from build123d import *

# Parameters (mm, degrees)
SKETCH1_W           = 56
SKETCH1_H           = 28
BOSS_EXTRUDE1_DEPTH = 16
SKETCH2_W           = 52
SKETCH2_H           = 24
CUT_EXTRUDE1_DEPTH  = 8
SKETCH3_W           = 24
SKETCH3_H           = 24
CUT_EXTRUDE2_DEPTH  = 2
SKETCH4_W           = 52
SKETCH4_H           = 2
CUT_EXTRUDE3_DEPTH  = 1
SKETCH5_R           = 6.75
CUT_EXTRUDE4_DEPTH  = 1
CUT_EXTRUDE5_REACH  = 7
SKETCH6_R           = 5
SKETCH7_R           = 6.75
CUT_EXTRUDE6_DEPTH  = 1
SKETCH8_R           = 6.75
CUT_EXTRUDE7_DEPTH  = 1
CUT_EXTRUDE8_DEPTH  = 26


with BuildPart() as part:
    # Sketch1 → Boss-Extrude1 (new body)
    with BuildSketch(Plane(origin=(0, 0, 0), x_dir=(1, 0, 0), z_dir=(0, 1, 0))):
        Rectangle(SKETCH1_W, SKETCH1_H)
    extrude(amount=BOSS_EXTRUDE1_DEPTH)

    # Sketch2 → Cut-Extrude1 (cut)
    with BuildSketch(Plane(origin=(0, 16, 0), x_dir=(1, 0, 0), z_dir=(0, 1, 0))):
        Rectangle(SKETCH2_W, SKETCH2_H)
    extrude(amount=-CUT_EXTRUDE1_DEPTH, mode=Mode.SUBTRACT)

    # Sketch3 → Cut-Extrude2 (cut)
    with BuildSketch(Plane(origin=(0, 8, 0), x_dir=(1, 0, 0), z_dir=(0, 1, 0))):
        Rectangle(SKETCH3_W, SKETCH3_H)
    extrude(amount=-CUT_EXTRUDE2_DEPTH, mode=Mode.SUBTRACT)

    # Sketch4 → Cut-Extrude3 (cut)
    with BuildSketch(Plane(origin=(0, 8, 0), x_dir=(1, 0, 0), z_dir=(0, 1, 0))):
        Rectangle(SKETCH4_W, SKETCH4_H)
    extrude(amount=-CUT_EXTRUDE3_DEPTH, mode=Mode.SUBTRACT)

    # Sketch5 → Cut-Extrude4 (cut)
    with BuildSketch(Plane(origin=(0, 6, 0), x_dir=(1, 0, 0), z_dir=(0, 1, 0))):
        Circle(SKETCH5_R)
    extrude(amount=-CUT_EXTRUDE4_DEPTH, mode=Mode.SUBTRACT)

    # Sketch6 → Cut-Extrude5 (cut, up to next)
    with BuildSketch(Plane(origin=(0, 5, 0), x_dir=(1, 0, 0), z_dir=(0, 1, 0)), mode=Mode.PRIVATE) as cut_extrude5_sk1:
        Circle(SKETCH6_R)
    cut_extrude5_tool1 = extrude(cut_extrude5_sk1.sketch, amount=-CUT_EXTRUDE5_REACH, mode=Mode.PRIVATE) & part.part
    add(cut_extrude5_tool1.solids().sort_by_distance((0, 5, 0))[0], mode=Mode.SUBTRACT)

    # Sketch7 → Cut-Extrude6 (cut)
    with BuildSketch(Plane.XY.offset(14)):
        with Locations((0, 8)):
            Circle(SKETCH7_R)
    extrude(amount=-CUT_EXTRUDE6_DEPTH, mode=Mode.SUBTRACT)

    # Sketch8 → Cut-Extrude7 (cut)
    with BuildSketch(Plane(origin=(0, 0, -14), x_dir=(-1, 0, 0), z_dir=(0, 0, -1))):
        with Locations((0, 8)):
            Circle(SKETCH8_R)
    extrude(amount=-CUT_EXTRUDE7_DEPTH, mode=Mode.SUBTRACT)

    # Sketch9 → Cut-Extrude8 (cut)
    with BuildSketch(Plane.XY.offset(13)):
        with BuildLine():
            Line((-4.582575695, 6), (4.582575695, 6))
            ThreePointArc((4.582575695, 6), (0, 13), (-4.582575695, 6))
        make_face()
    extrude(amount=-CUT_EXTRUDE8_DEPTH, mode=Mode.SUBTRACT)

    # Sketch11 → Cut-Revolve2 (revolve, cut)
    with BuildSketch(Plane(origin=(0, 0, 0), x_dir=(0, 0, -1), z_dir=(1, 0, 0))):
        Polygon((0, 0), (-10, 0), (0, 10), align=None)
    revolve(axis=Axis((0, 10, 0), (0, -1, 0)), mode=Mode.SUBTRACT)


solid = part.part
Design review of the part built by this model. Coordinates are the model's own, in mm. A direction names the side the tool comes from. Give positions to 0.01 mm unless a question says otherwise; leave off trailing zeros. Order: outer loops, then holes, each group sorted by start corner. A loop starts at its lowest first (then second) coordinate and runs counter-clockwise, first axis right, second up. Notation, with made-up numbers: (-24.5, 81) - (17.5, 81) arc R25 cw to (17.5, 95) - close; hole circle Ø7 at (46.25, 52). An arc over 180 degrees is marked (long way). Write item = value, one per line. Start each with the question number.
Q1. Tool access review of faces 5 (the face through (-26, 12, 0)), 6 (the face through (0.879, 14.693, -13.507)), 7 (the face through (0.1, 13, -12.5)), 8 (the face through (-0.879, 14.693, 13.507)): name each direction out of +Z, -Z, +X, -X, +Y, -Y from which nothing blocks a thin tool from reaching the whole face with its end or side.
Q2. We need section A-A on z = 0. State the section outline as (x, y) points, plus the area to 4 significant figures.
Q3. Clearance check with flat-ended pins moving along their axes: pin 1 Ø2 at (x, z) = (12.5, -7.5) entering from +Y; pin 2 Ø8 at (x, y) = (0, 8) entering from -Z; pin 3 Ø0.6 at (x, z) = (-21, 0) entering from +Y. State where each tip first meets the part, or that it passes through.
Q4. To check wall thickness, follow L1, parallel to X at y = 10, z = -9.5; L2, parallel to Z at x = 25, y = 11; L3, parallel to Y at x = 0, z = 13.6. State the ranges of each line that lie inside material, in increasing order. Write a range as from..to.
Q5. Mouldability with a two-part tool opening along Z and no side actions: class faces 1 (the face through (-28, 8, 0)), 2 (the face through (-0.4, 13.3, 12)), 3 (the face through (-19.1, 7.5, 1)), 4 (the face through (0, 5, -13)) as released by +Z, released by -Z, zero draft, split by the parting line, or undercut.
Q6. We need section C-C on x = 0. State the section outline as (y, z) points, plus the area to 3 significant figures.
Q7. We need section D-D on y = 11.25. State the section outline as (x, z) points, plus the area to 3 significant figures.
Q8. We need section B-B on x = 19. State the section outline as (y, z) points, plus the area to 3 significant figures.
Working result:
q1.face_5 = +Y
q1.face_6 = -Z
q1.face_7 = +Z, -Z
q1.face_8 = +Z
q2.outline = (-28, 0) - (-10, 0) - (-5, 5) - (-6.75, 5) - (-6.75, 6) - (-12, 6) - (-12, 7) - (-26, 7) - (-26, 16) - (-28, 16) - close; (5, 5) - (10, 0) - (28, 0) - (28, 16) - (26, 16) - (26, 7) - (12, 7) - (12, 6) - (6.75, 6) - (6.75, 5) - close
q2.area = 315.5 mm²
q3.pin_1 = 8
q3.pin_2 = -13
q3.pin_3 = 7
q4.L1 = -28..-26, 26..28
q4.L2 = -14..-12, 12..14
q4.L3 = 0..1.25, 14.75..16
q5.face_1 = zero draft
q5.face_2 = undercut
q5.face_3 = undercut
q5.face_4 = released by -Z
q6.outline = (0, -14) - (1.25, -14) - (1.25, -13) - (6, -13) - (6, -6.75) - (5, -6.75) - (5, -5) - (0, -10) - close; (0, 10) - (5, 5) - (5, 6.75) - (6, 6.75) - (6, 13) - (1.25, 13) - (1.25, 14) - (0, 14) - close; (13, -13) - (14.75, -13) - (14.75, -14) - (16, -14) - (16, -12) - (13, -12) - close; (13, 12) - (16, 12) - (16, 14) - (14.75, 14) - (14.75, 13) - (13, 13) - close
q6.area = 78.5 mm²
q7.outline = (-28, -14) - (-5.92, -14) - (-5.92, -13) - (-3.8, -13) - (-3.8, -12) - (-26, -12) - (-26, 12) - (-3.8, 12) - (-3.8, 13) - (-5.92, 13) - (-5.92, 14) - (-28, 14) - close; (3.8, -13) - (5.92, -13) - (5.92, -14) - (28, -14) - (28, 14) - (5.92, 14) - (5.92, 13) - (3.8, 13) - (3.8, 12) - (26, 12) - (26, -12) - (3.8, -12) - close
q7.area = 281 mm²
q8.outline = (0, -14) - (16, -14) - (16, -12) - (8, -12) - (8, -1) - (7, -1) - (7, 1) - (8, 1) - (8, 12) - (16, 12) - (16, 14) - (0, 14) - close
q8.area = 254 mm²
